```python
from build123d import *

# Parameters (mm, degrees)
BOSS_EXTRUDE1_DEPTH = 3.2


with BuildPart() as part:
    # Sketch1 → Boss-Extrude1 (new body)
    with BuildSketch(Plane.XY):
        Polygon((0, 4.041451884), (-3.5, 2.020725942), (-3.5, -2.020725942), (0, -4.041451884), (3.5, -2.020725942), (3.5, 2.020725942), align=None)
    extrude(amount=-BOSS_EXTRUDE1_DEPTH)

    # Sketch4 → Cut-Revolve1 (revolve, cut)
    with BuildSketch(Plane(origin=(0, 0, 0), x_dir=(0, 0, -1), z_dir=(1, 0, 0))):
        Polygon((3.2, 4.041451884), (2.540982447, 4.041451884), (3.2, 2.9), align=None)
        Polygon((0, 4.041451884), (0.659017553, 4.041451884), (0, 2.9), align=None)
    revolve(axis=Axis((0, 0, 0), (0, 0, -1)), mode=Mode.SUBTRACT)

    # Sketch5 → Cut-Revolve2 (revolve, cut)
    with BuildSketch(Plane(origin=(0, 0, 0), x_dir=(0, 0, -1), z_dir=(1, 0, 0))):
        Polygon((0, 0), (0, 2.05), (0.230940108, 1.65), (2.969059892, 1.65), (3.2, 2.05), (3.2, 0), align=None)
    revolve(axis=Axis((0, 0, 0), (0, 0, -1)), mode=Mode.SUBTRACT)


solid = part.part
```
The model under review builds one solid part; all positions refer to its coordinate system, in mm. Coordinates: 2 decimals unless noted, no trailing zeros. Write each loop counter-clockwise with the first axis right and the second up, starting at its lowest first coordinate (ties: lowest second). Pieces come first, ordered by that corner, then holes. Notation, with made-up numbers: (17, -14.5) - (26, -14.5) arc R23 cw to (26, 20.5) - close; hole circle Ø11 at (72.25, 15). An arc over 180 degrees is marked (long way). Answer in a Markdown table with one row per item. Add a question column.
Q1. Consider section B-B on z = -2.3. Give the boundary of the cut face in (x, y), then the cut area to 3 significant figures.
Q2. Consider section A-A on y = 0. Give the boundary of the cut face in (x, z), then the cut area to 3 significant figures.
Q3. Clearance check with flat-ended pins moving along their axes: pin 1 (1 mm diameter, centred on x = -1, z = -2, fed in from -Y); pin 2 (1.5 mm diameter, centred on x = 1, z = -0.5, fed in from +Y). State where each tip first meets the part, or that it passes through.
Q4. To check wall thickness, follow line 1 along X through (y, z) = (0, -0.95); line 2 along Y through (x, z) = (0.25, -0.3); line 3 along X through (y, z) = (1.5, -0.4). State the ranges of each line that lie inside material, in increasing order. Write a range as from..to.
Q5. Draft analysis for pull direction X (two halves, no side actions). For faces 1 (the face through (1.115, -1.216, -1.619)), 2 (the face through (-1.726, 3.045, -1.582)), 3 (the face through (1, 2, 0)), state which applies: +X half, -X half, draft (parallel to the pull), parting line (faces both ways), or undercut.
Answers below:
| question | item | result |
|---|---|---|
| 1 | outline | (-3.5, -2.02) - (0, -4.04) - (3.5, -2.02) - (3.5, 2.02) - (0, 4.04) - (-3.5, 2.02) - close; hole circle Ø3.3 at (0, 0) |
| 1 | area | 33.9 mm² |
| 2 | outline | (-3.5, -2.85) - (-2.9, -3.2) - (-2.05, -3.2) - (-1.65, -2.97) - (-1.65, -0.23) - (-2.05, 0) - (-2.9, 0) - (-3.5, -0.35) - close; (1.65, -2.97) - (2.05, -3.2) - (2.9, -3.2) - (3.5, -2.85) - (3.5, -0.35) - (2.9, 0) - (2.05, 0) - (1.65, -0.23) - close |
| 2 | area | 11.2 mm² |
| 3 | pin 1 | y = -3.75 |
| 3 | pin 2 | y = 3.89 |
| 4 | line 1 | -3.5..-1.65, 1.65..3.5 |
| 4 | line 2 | -3.41..-1.63, 1.63..3.41 |
| 4 | line 3 | -3.26..-0.69, 0.69..3.26 |
| 5 | face 1 | undercut |
| 5 | face 2 | -X half |
| 5 | face 3 | draft |
